```python
from build123d import *

# Parameters (mm, degrees)
SKETCH_1_W          = 40
SKETCH_1_H          = 37
EXTRUDE_1_DEPTH     = 51
SKETCH_3_W          = 33
SKETCH_3_H          = 47
CUT_EXTRUDE_2_DEPTH = 38
CUT_EXTRUDE_3_REACH = 59.821
SKETCH_4_W          = 10
SKETCH_4_H          = 33
CUT_EXTRUDE_4_REACH = 59.821
SKETCH_5_W          = 7
SKETCH_5_H          = 17
CUT_EXTRUDE_5_REACH = 59.821
SKETCH_6_R          = 1.1
SKETCH_7_W          = 37
SKETCH_7_H          = 5
EXTRUDE_2_DEPTH     = 40
SKETCH_9_R          = 1.6
SKETCH_9_R_2        = 1.1
CUT_EXTRUDE_6_DEPTH = 5
CUT_EXTRUDE_7_REACH = 68.106
SKETCH_12_R         = 1.6
FILLET_1_R          = 1


with BuildPart() as part:
    # 草图1 → 凸台-拉伸1 (new body)
    with BuildSketch(Plane(origin=(0, 0, 0), x_dir=(1, 0, 0), z_dir=(0, 1, 0))):
        Rectangle(SKETCH_1_W, SKETCH_1_H)
    extrude(amount=EXTRUDE_1_DEPTH)

    # 草图3 → 切除-拉伸2 (cut)
    with BuildSketch(Plane.ZY.offset(20)):
        with Locations((0, 25.5)):
            Rectangle(SKETCH_3_W, SKETCH_3_H)
    extrude(amount=-CUT_EXTRUDE_2_DEPTH, mode=Mode.SUBTRACT)

    # 草图4 → 切除-拉伸3 (cut, up to next)
    with BuildSketch(Plane(origin=(0, 51, 0), x_dir=(1, 0, 0), z_dir=(0, 1, 0)), mode=Mode.PRIVATE) as cut_extrude_3_sk1:
        with Locations((13, 0)):
            Rectangle(SKETCH_4_W, SKETCH_4_H)
    cut_extrude_3_tool1 = extrude(cut_extrude_3_sk1.sketch, amount=-CUT_EXTRUDE_3_REACH, mode=Mode.PRIVATE) & part.part
    add(cut_extrude_3_tool1.solids().sort_by_distance((13, 51, 0))[0], mode=Mode.SUBTRACT)

    # 草图5 → 切除-拉伸4 (cut, up to next)
    with BuildSketch(Plane(origin=(0, 51, 0), x_dir=(1, 0, 0), z_dir=(0, 1, 0)), mode=Mode.PRIVATE) as cut_extrude_4_sk1:
        with Locations((-16.5, 0)):
            Rectangle(SKETCH_5_W, SKETCH_5_H)
    cut_extrude_4_tool1 = extrude(cut_extrude_4_sk1.sketch, amount=-CUT_EXTRUDE_4_REACH, mode=Mode.PRIVATE) & part.part
    add(cut_extrude_4_tool1.solids().sort_by_distance((-16.5, 51, 0))[0], mode=Mode.SUBTRACT)

    # 草图6 → 切除-拉伸5 (cut, up to next)
    with BuildSketch(Plane(origin=(0, 51, 0), x_dir=(1, 0, 0), z_dir=(0, 1, 0)), mode=Mode.PRIVATE) as cut_extrude_5_sk1:
        with Locations(Location((-18, 10.75, 0), (0, 0, 270))):
            Circle(SKETCH_6_R)
    cut_extrude_5_tool1 = extrude(cut_extrude_5_sk1.sketch, amount=-CUT_EXTRUDE_5_REACH, mode=Mode.PRIVATE) & part.part
    # 草图6 → 切除-拉伸5 (cut, up to next)
    with BuildSketch(Plane(origin=(0, 51, 0), x_dir=(1, 0, 0), z_dir=(0, 1, 0)), mode=Mode.PRIVATE) as cut_extrude_5_sk2:
        with Locations(Location((-18, -10.75, 0), (0, 0, 270))):
            Circle(SKETCH_6_R)
    cut_extrude_5_tool2 = extrude(cut_extrude_5_sk2.sketch, amount=-CUT_EXTRUDE_5_REACH, mode=Mode.PRIVATE) & part.part
    # 草图6 → 切除-拉伸5 (cut, up to next)
    with BuildSketch(Plane(origin=(0, 51, 0), x_dir=(1, 0, 0), z_dir=(0, 1, 0)), mode=Mode.PRIVATE) as cut_extrude_5_sk3:
        with Locations(Location((4, 10.75, 0), (0, 0, 270))):
            Circle(SKETCH_6_R)
    cut_extrude_5_tool3 = extrude(cut_extrude_5_sk3.sketch, amount=-CUT_EXTRUDE_5_REACH, mode=Mode.PRIVATE) & part.part
    # 草图6 → 切除-拉伸5 (cut, up to next)
    with BuildSketch(Plane(origin=(0, 51, 0), x_dir=(1, 0, 0), z_dir=(0, 1, 0)), mode=Mode.PRIVATE) as cut_extrude_5_sk4:
        with Locations(Location((4, -10.75, 0), (0, 0, 270))):
            Circle(SKETCH_6_R)
    cut_extrude_5_tool4 = extrude(cut_extrude_5_sk4.sketch, amount=-CUT_EXTRUDE_5_REACH, mode=Mode.PRIVATE) & part.part
    add(cut_extrude_5_tool1.solids().sort_by_distance((-18, 51, -10.75))[0], mode=Mode.SUBTRACT)
    add(cut_extrude_5_tool2.solids().sort_by_distance((-18, 51, 10.75))[0], mode=Mode.SUBTRACT)
    add(cut_extrude_5_tool3.solids().sort_by_distance((4, 51, -10.75))[0], mode=Mode.SUBTRACT)
    add(cut_extrude_5_tool4.solids().sort_by_distance((4, 51, 10.75))[0], mode=Mode.SUBTRACT)

    # 草图7 → 凸台-拉伸2 (add)
    with BuildSketch(Plane.ZY.offset(20)):
        with Locations((0, -2.5)):
            Rectangle(SKETCH_7_W, SKETCH_7_H)
    extrude(amount=-EXTRUDE_2_DEPTH)

    # 草图9 → 切除-拉伸6 (cut)
    with BuildSketch(Plane.ZY.offset(20)):
        with Locations((-10, -2)):
            Circle(SKETCH_9_R)
        with Locations(Location((10, -2, 0), (0, 0, 180))):
            Circle(SKETCH_9_R)
        with Locations((-15.5, -2)):
            Circle(SKETCH_9_R_2)
        with Locations(Location((15.5, -2, 0), (0, 0, 180))):
            Circle(SKETCH_9_R_2)
    extrude(amount=-CUT_EXTRUDE_6_DEPTH, mode=Mode.SUBTRACT)

    # 切除-拉伸7: up to this face of the body (flat: up to its plane)
    cut_extrude_7_end = Plane(part.part.faces().sort_by_distance((0, 23, 18.5))[0])
    # 草图12 → 切除-拉伸7 (cut, up to the picked face)
    with BuildSketch(Plane(origin=(0, 0, -18.5), x_dir=(-1, 0, 0), z_dir=(0, 0, -1)), mode=Mode.PRIVATE) as cut_extrude_7_sk1:
        with Locations((17, 41)):
            Circle(SKETCH_12_R)
    cut_extrude_7_tool1 = split(extrude(cut_extrude_7_sk1.sketch, amount=-CUT_EXTRUDE_7_REACH, mode=Mode.PRIVATE), bisect_by=cut_extrude_7_end, keep=Keep.BOTH, mode=Mode.PRIVATE)
    # 草图12 → 切除-拉伸7 (cut, up to the picked face)
    with BuildSketch(Plane(origin=(0, 0, -18.5), x_dir=(-1, 0, 0), z_dir=(0, 0, -1)), mode=Mode.PRIVATE) as cut_extrude_7_sk2:
        with Locations((17, 31)):
            Circle(SKETCH_12_R)
    cut_extrude_7_tool2 = split(extrude(cut_extrude_7_sk2.sketch, amount=-CUT_EXTRUDE_7_REACH, mode=Mode.PRIVATE), bisect_by=cut_extrude_7_end, keep=Keep.BOTH, mode=Mode.PRIVATE)
    add(cut_extrude_7_tool1.solids().sort_by(Axis((-17, 41, -18.5), (0, 0, 1)))[0], mode=Mode.SUBTRACT)
    add(cut_extrude_7_tool2.solids().sort_by(Axis((-17, 31, -18.5), (0, 0, 1)))[0], mode=Mode.SUBTRACT)

    # 圆角1
    fillet_1_edges = [part.edges().sort_by_distance(p)[0] for p in [
        (0, 51, 18.5),
        (0, -5, -18.5),
        (0, -5, 18.5),
        (0, 51, -18.5),
    ]]
    fillet(fillet_1_edges, radius=FILLET_1_R)


solid = part.part
```
Part model, mm, in its own coordinate system. A direction names the side the tool comes from. Round coordinates to 2 decimals unless told otherwise and drop trailing zeros. Loops run counter-clockwise (first coordinate to the right, second up) from the corner with the lowest first, then second, coordinate; pieces in that order, holes last. Notation, with made-up numbers: (11, 71.25) -> (23, 71.25) arc R24 cw to (23, 91.25) -> close; hole circle Ø8 at (47.25, 6). An arc over 180 degrees is marked (long way). Use a Markdown table: item, result.
1) Tool access for faces 1 (the flat face through (-17, 50, 8.5)), 2 (the cylindrical face through (4.93, 50.01, 11.34)), 3 (the flat face through (-15, -2, -16)): list every direction of +Z, -Z, +X, -X, +Y, -Y with a clear straight run to the whole face (end or side of a thin tool).
The answers:
| item | result |
|---|---|
| face 1 | -X, +Y |
| face 2 | +Y |
| face 3 | -X |
2) Cut at C-C, the plane x = -11.5. List the corners of the cut face in (y, z), and give its area (3 significant figures).
The answers:
| item | result |
|---|---|
| outline | (-5, -17.5) arc R1 ccw to (-4, -18.5) -> (50, -18.5) arc R1 ccw to (51, -17.5) -> (51, 17.5) arc R1 ccw to (50, 18.5) -> (-4, 18.5) arc R1 ccw to (-5, 17.5) -> close; hole (2, -16.5) -> (49, -16.5) -> (49, 16.5) -> (2, 16.5) -> close |
| area | 520 mm2 |
3) Probe line 1 (Y direction, x = -16, z = -10); line 2 (X direction, y = 49.9, z = -10.75); line 3 (Y direction, x = 4, z = 12). List the from-to ranges inside material, lowest first. Write a range as [from, to].
The answers:
| item | result |
|---|---|
| line 1 | y = [-5, -3.6], [-0.4, 2], [49, 51] |
| line 2 | x = [-20, -19.1], [-16.9, 2.9], [5.1, 8], [18, 20] |
| line 3 | y = [-5, 2], [49, 51] |
4) Pull direction X, two halves, no side cores. Call faces 4 (the cylindrical face through (-17.54, -1.93, -11.6)), 5 (the cylindrical face through (-15.73, 40.03, -17.51)), 6 (the flat face through (20, 23, 0)): pulls with the +X half, pulls with the -X half, needs draft (parallel to the pull), parting line crosses it, or undercut.
The answers:
| item | result |
|---|---|
| face 4 | needs draft |
| face 5 | undercut |
| face 6 | pulls with the +X half |
5) Cut at B-B, the plane y = 41. List the corners of the cut face in (x, z).
The answers:
| item | result |
|---|---|
| outline | (-20, -18.5) -> (-18.6, -18.5) -> (-18.6, -16.5) -> (-20, -16.5) -> close; (-20, 16.5) -> (-18.6, 16.5) -> (-18.6, 18.5) -> (-20, 18.5) -> close; (-15.4, -18.5) -> (20, -18.5) -> (20, 18.5) -> (-15.4, 18.5) -> (-15.4, 16.5) -> (18, 16.5) -> (18, -16.5) -> (-15.4, -16.5) -> close |
6) Drop flat-ended pins along their axis: pin 1 Ø2.5 at (y, z) = (-2, 10) entering from -X; pin 2 Ø16.5 at (y, z) = (34.5, -1) entering from -X; pin 3 Ø1.3 at (x, z) = (-18, -10.75) entering from +Y; pin 4 Ø2.5 at (y, z) = (-2.5, 10.5) entering from -X. Give the stop position or say it passes through.
The answers:
| item | result |
|---|---|
| pin 1 | stops at x = -15 |
| pin 2 | stops at x = 18 |
| pin 3 | stops at y = 2 |
| pin 4 | stops at x = -20 |
7) Cut at A-A, the plane z = 15.5. List the corners of the cut face in (x, y).
The answers:
| item | result |
|---|---|
| outline | (-20, -5) -> (20, -5) -> (20, 51) -> (18, 51) -> (18, 2) -> (-20, 2) -> (-20, -0.9) -> (-15, -0.9) -> (-15, -3.1) -> (-20, -3.1) -> close; (-20, 49) -> (8, 49) -> (8, 51) -> (-20, 51) -> close |
8) Cut at D-D, the plane x = 4. List the corners of the cut face in (y, z).
The answers:
| item | result |
|---|---|
| outline | (-5, -17.5) arc R1 ccw to (-4, -18.5) -> (50, -18.5) arc R1 ccw to (51, -17.5) -> (51, -11.85) -> (49, -11.85) -> (49, -16.5) -> (2, -16.5) -> (2, 16.5) -> (49, 16.5) -> (49, 11.85) -> (51, 11.85) -> (51, 17.5) arc R1 ccw to (50, 18.5) -> (-4, 18.5) arc R1 ccw to (-5, 17.5) -> close; (49, -9.65) -> (51, -9.65) -> (51, 9.65) -> (49, 9.65) -> close |
